```python
from build123d import *

# Parameters (mm, degrees)
BOSS_EXTRUDE1_DEPTH     = 3.81
CUT_EXTRUDE1_DEPTH      = 108.860315687
CUT_EXTRUDE1_DEPTH_BACK = 108.860315687
FILLET3_START           = -1
FILLET3_DEPTH           = 6
FILLET3_2_DEPTH         = 3.81


with BuildPart() as part:
    # Sketch1 → Boss-Extrude1 (new body)
    with BuildSketch(Plane(origin=(0, 0, 0), x_dir=(0, 0, -1), z_dir=(1, 0, 0))):
        Polygon((-88.9, 3.81), (-63.5, 3.81), (-63.5, 0), (-38.1, 0), (-38.1, 3.81), (-26.9875, 3.81), (-26.9875, 6.35), (-28.5242, 6.35), (-28.5242, 8.763), (-26.9875, 8.763), (-26.9875, 12.954), (-23.8125, 12.954), (-23.8125, 8.763), (-22.2758, 8.763), (-22.2758, 6.35), (-23.8125, 6.35), (-23.8125, 3.81), (-12.7, 3.81), (-12.7, 0), (12.7, 0), (12.7, 3.81), (23.8125, 3.81), (23.8125, 6.35), (22.2758, 6.35), (22.2758, 8.763), (23.8125, 8.763), (23.8125, 12.954), (26.9875, 12.954), (26.9875, 8.763), (28.5242, 8.763), (28.5242, 6.35), (26.9875, 6.35), (26.9875, 3.81), (38.1, 3.81), (38.1, 0), (63.5, 0), (63.5, 3.81), (74.6125, 3.81), (74.6125, 6.35), (73.0758, 6.35), (73.0758, 8.763), (74.6125, 8.763), (74.6125, 12.954), (77.7875, 12.954), (77.7875, 8.763), (79.3242, 8.763), (79.3242, 6.35), (77.7875, 6.35), (77.7875, 3.81), (88.9, 3.81), (69.85, 60.96), (57.15, 60.96), (57.15, 57.15), (46.0375, 57.15), (46.0375, 54.61), (47.5742, 54.61), (47.5742, 52.197), (46.0375, 52.197), (46.0375, 48.006), (42.8625, 48.006), (42.8625, 52.197), (41.3258, 52.197), (41.3258, 54.61), (42.8625, 54.61), (42.8625, 57.15), (31.75, 57.15), (31.75, 60.96), (19.05, 60.96), (19.05, 57.15), (7.9375, 57.15), (7.9375, 54.61), (9.4742, 54.61), (9.4742, 52.197), (7.9375, 52.197), (7.9375, 48.006), (4.7625, 48.006), (4.7625, 52.197), (3.2258, 52.197), (3.2258, 54.61), (4.7625, 54.61), (4.7625, 57.15), (-6.35, 57.15), (-6.35, 60.96), (-19.05, 60.96), (-88.9, 16.51), align=None)
    extrude(amount=BOSS_EXTRUDE1_DEPTH)

    # Sketch2 → Cut-Extrude1 (cut, two sides: drawn at the far end of the back side and taken through both)
    with BuildSketch(Plane(origin=(0, 0, 0), x_dir=(0, 0, -1), z_dir=(1, 0, 0)).offset(-CUT_EXTRUDE1_DEPTH_BACK)):
        Polygon((-37.957173184, 48.928162519), (-88.9, 16.51), (-19.05, 16.51), (-19.05, 60.96), align=None)
    extrude(amount=CUT_EXTRUDE1_DEPTH + CUT_EXTRUDE1_DEPTH_BACK, mode=Mode.SUBTRACT)

    # Fillet3: read off the stored shape, not the designer's step
    # Fillet3 outline → Fillet3 (cut)
    with BuildSketch(Plane.YZ.offset(FILLET3_START)):
        with BuildLine():
            ThreePointArc((3.81, 88.9), (12.790256121, 85.180256121), (16.51, 76.2))
            Line((16.51, 76.2), (16.51, 88.9))
            Line((16.51, 88.9), (3.81, 88.9))
        make_face()
    extrude(amount=FILLET3_DEPTH, mode=Mode.SUBTRACT)

    # Fillet3 2 outline → Fillet3 2 (add)
    with BuildSketch(Plane.YZ):
        with BuildLine():
            ThreePointArc((29.21, 19.05), (20.229743879, 22.769743879), (16.51, 31.75))
            Line((16.51, 31.75), (16.51, 19.05))
            Line((16.51, 19.05), (29.21, 19.05))
        make_face()
    extrude(amount=FILLET3_2_DEPTH)


solid = part.part
```
Here's how the part is built. I have some questions about the finished solid (model axes, mm). A direction names the side the tool comes from. Coordinates: 2 decimals unless noted, no trailing zeros. Loops run counter-clockwise (first coordinate to the right, second up) from the corner with the lowest first, then second, coordinate; pieces in that order, holes last. Notation, with made-up numbers: (58.5, -33) - (63.5, -33) arc R12 cw to (63.5, -16) - close; hole circle Ø3 at (-35.75, 4.5). An arc over 180 degrees is marked (long way). Return JSON: item names as keys, results as strings. Group by question number.
Item 1: Will these pins go through, and if not, where does the flat tip stop? P1, Ø2, axis at x = 2.5, z = 5, coming from the +Y side; P2, Ø1.9, axis at x = 2.5, y = 2.5, coming from the -Z side; P3, Ø0.5, axis at x = 1, z = -4, coming from the -Y side; P4, Ø1, axis at x = 2, y = 45.5, coming from the -Z side.
Item 2: I need wall thicknesses on line 1 (Z direction, x = 2.9, y = 49); line 2 (Z direction, x = 0.5, y = 56); line 3 (Z direction, x = 2.4, y = 9.5). Which ranges of each line are inside material? Lowest first, please. Write a range as from..to.
Item 3: We'd pull the mould along Z, two halves only. Please class faces 4 (the face through (2, 2, 12.7)), 5 (the face through (2, 60.96, 13)), 6 (the face through (1.88, 31.98, -79.51)): +Z half, -Z half, draft (parallel to the pull), parting line (faces both ways), or undercut.
Item 4: If we section it at B-B on z = -54: Write out the boundary of the cut face in (x, y), and give its area (3 significant figures).
Item 5: If we section it at A-A on y = 36: Write out the boundary of the cut face in (x, z), and give its area (3 significant figures).
Item 6: On a 3-axis mill with a long thin cutter (end or side, diameter ignored), from which of +Z, -Z, +X, -X, +Y, -Y can I reach the whole of each face in a straight line? I mean faces 1 (the face through (2, 50, -46.038)), 2 (the face through (2, 11, -77.788)), 3 (the face through (2, 45, 19.05)). Say none if no direction works.
Calculated:
{
 "1": {"P1": "stops at y = 57.15", "P2": "stops at z = -63.5", "P3": "stops at y = 0", "P4": "stops at z = -75.17"},
 "2": {"line 1": "z = -73.84..-46.04, -42.86..-7.94, -4.76..19.05", "line 2": "z = -71.5..-46.04, -42.86..-7.94, -4.76..19.05", "line 3": "z = -87..-77.79, -74.61..-26.99, -23.81..23.81, 26.99..87.55"},
 "3": {"face 4": "undercut", "face 5": "draft", "face 6": "-Z half"},
 "4": {"outline": "(0, 0) - (3.81, 0) - (3.81, 57.15) - (0, 57.15) - close", "area": "218 mm^2"},
 "5": {"outline": "(0, -78.17) - (3.81, -78.17) - (3.81, 19.05) - (0, 19.05) - close", "area": "370 mm^2"},
 "6": {"face 1": "+X, -X, +Y", "face 2": "+X, -X, -Y", "face 3": "+Z, +X, -X, +Y"}
}
